Autodesk Inventor part; units mm, degrees
ref_plane "YZ Plane" through (0, 0, 0) normal (1, 0, 0) x (0, 1, 0)
ref_plane "XZ Plane" through (0, 0, 0) normal (0, 1, 0) x (-1, 0, 0)
ref_plane "XY Plane" through (0, 0, 0) normal (0, 0, 1) x (1, 0, 0)
sketch "Sketch1" plane through (0, 0, 0) normal (0, 1, 0) x (-1, 0, 0)
  line L0 (0, 0) -> (-2, 0)
  line L1 (-2, 0) -> (-4, 0)
  line L2 (0, 0) -> (0, -15)
  line L3 (0, -15) -> (0, -25)
  circle A0 centre (0, -25) radius 10
  line L4 (-1.5, -15.1131) -> (0, -15.1131)
  line L5 (0, -15.1131) -> (0, -15)
  line L6 (-1.5, -15) -> (-1.5, -15.1131)
  line L7 (-1.5, -15.1131) -> (-2, 0)
  line L8 (0, -15) -> (-1.5, -15)
  line L9 (-1.5, -15) -> (-2, -15)
  line L10 (-2, -15) -> (-2, -15.202)
  line L11 (-2, -15.202) -> (-4, 0)
  line L12 (0, -25) -> (0, -35)
  circle A1 centre (0, -25) radius 9.2
  line L13 (-1.5, -15.1131) -> (-1.4733, -15.9187)
  point P0 (0, -34.2)
  dimension "d7" = 18.4
  dimension "d2" = 15
  dimension "d4" = 10
  dimension "d6" = 0.5
  dimension "d10" = 1.5
  dimension "d11" = 2
  dimension "d12" = 2
revolve "Revolution1" add sketch "Sketch1" angle 180 about axis through (0, 0, 0) along (0, 0, 1) contours L7 L9 L10 L11 L1 | L7 A0 L10 L9 | L13 A1 L12 A0
sketch "Sketch2" plane through (0, 0, 0) normal (0, 0, 1) x (1, 0, 0)
  line L0 (5, 0) -> (-5, 0)
  line L1 (-14, 0) -> (14, 0)
  arc A0 (2, 0) -> (-2, 0) centre (0, 0) ccw
  line L2 (0, 0) -> (0, 16) construction
  line L3 (-10, 0) -> (10, 0)
  line L4 (10, 0) -> (10, 15)
  line L5 (10, 15) -> (-10, 15)
  line L6 (-10, 15) -> (-10, 0)
  point P0 (0, 0)
  point P1 (0, 0)
  point P2 (-10, 0)
  point P3 (10, 0)
  dimension "d29" = 20
  dimension "d33" = 15
  dimension "d34" = 15
extrude "Base" add sketch "Sketch2" along normal blind 7 contours L0 A0 L1 L6 L5 L4
sketch "Sketch3" plane through (0, 0, 0) normal (0, 0, -1) x (-1, 0, 0)
  line L0 (0, -3) -> (0, 18)
  line L1 (-10, 15) -> (10, 15)
  point P0 (0, 0)
  point P1 (0, 9.5)
  dimension "d30" = 5.5
hole "Screw Hole" at (0, 9.5, 0) direction (0, 0, 1) diameter 4.2 end through all counterbore diameter 8 counterbore depth 3
sketch "Sketch4" plane through (0, 0, 0) normal (0, 0, -1) x (-1, 0, 0)
  line L0 (-2, 0) -> (-10, 0)
  line L1 (0, 0) -> (0, -2) construction
  line L2 (6, 0) -> (6, 6)
  line L3 (6, 6) -> (8, 6)
  line L4 (6, 6) -> (4, 6)
  line L5 (4, 6) -> (5, 0)
  line L6 (7, 0) -> (8, 6)
  line L7 (7, 0) -> (5, 0)
  line L8 (10, 0) -> (2, 0)
  line L9 (6, 0) -> (6, 4)
  line L10 (7.6667, 4) -> (4.3333, 4)
  line L11 (0, 0) -> (0, 18)
  line L12 (10, 0) -> (4, 0)
  line L13 (-6, 0) -> (-6, 6)
  line L14 (-6, 6) -> (-8, 6)
  line L15 (-6, 6) -> (-4, 6)
  line L16 (-4, 6) -> (-5, 0)
  line L17 (-7, 0) -> (-8, 6)
  line L18 (-7, 0) -> (-5, 0)
  line L19 (-6, 0) -> (-6, 4)
  line L20 (-7.6667, 4) -> (-4.3333, 4)
  point P0 (5, 0)
  point P1 (-5, 0)
  point P2 (-5, 0)
extrude "Keyway" cut sketch "Sketch4" against normal through all contours L0 L13 L20 L16 | L0 L17 L20 L13 | L7 L5 L10 L2 | L2 L10 L6 L7
sketch "Sketch5" plane through (10, 0, 0) normal (1, 0, 0) x (0, 0, -1)
  line L0 (0, 15) -> (-7, 15)
  line L1 (0, 15) -> (-7, 15)
  line L2 (0, 0) -> (-7, 0)
  line L3 (-7, 15) -> (-7, 0)
  line L4 (-7, 15) -> (-7, 0)
  line L5 (-7, 0) -> (-6.5, 0)
  line L6 (-7, 15) -> (-6.5, 0)
  dimension "d37" = 0.5
extrude "Taper" cut sketch "Sketch5" against normal through all
fillet "Fillet1" radius 1 3 edges at (-10, 7.5, 0) (0, 15, 0) (10, 7.5, 0)
equation "\"d34\" = d33"
properties part number "markerWithRodEnd_3DPrint"
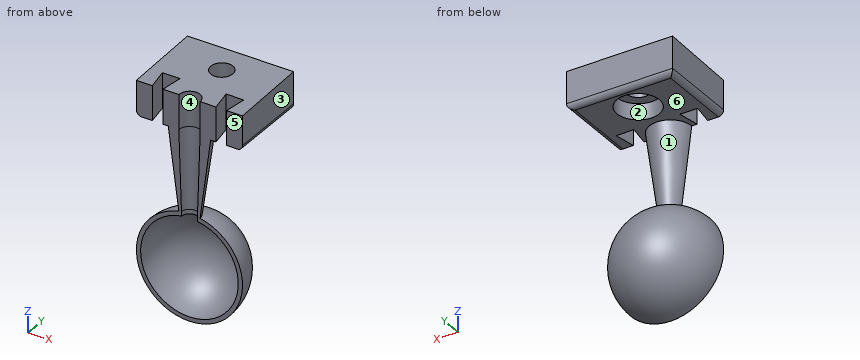
Design review of the part built by this model. Coordinates are the model's own, in mm. Face numbers are marked on the shaded views. A direction names the side the tool comes from. Give positions to 0.01 mm unless a question says otherwise; leave off trailing zeros. Loops run counter-clockwise (first coordinate to the right, second up) from the corner with the lowest first, then second, coordinate; pieces in that order, holes last. Notation, with made-up numbers: (76.5, 69) - (100.5, 69) arc R26 cw to (100.5, 83) - close; hole circle Ø1 at (66, 72). An arc over 180 degrees is marked (long way). Use CSV: the item, a comma, the result in double quotes. Start each with the question number.
1. Add section B-B (y = 12.5). State the section outline as (x, z) points, plus the area to 3 significant figures.
2. Machinability: for the marked faces 1, 2, 3 and 4, which of the approach directions +Z, -Z, +X, -X, +Y, -Y give a long, thin tool a straight path to every point of the face, cutting with its end or side? Answer none if there is none.
3. Draft analysis for pull direction Z (two halves, no side actions). For the marked faces 5 and 6, state which applies: released by +Z, released by -Z, zero draft, split by the parting line, or undercut.
4. Add section D-D (z = -27.5). State the section outline as (x, y) points, plus the area to 3 significant figures.
5. Add section C-C (z = 4). State the section outline as (x, y) points.
6. Add section A-A (x = 0). State the section outline as (y, z) points, plus the area to 3 significant figures.
7. Insertion check: P1, Ø6.5, axis at x = 0, y = 9.5, coming from the -Z side; P2, Ø3, axis at x = 1.5, y = 6, coming from the -Z side; P3, Ø6.5, axis at x = 0, y = 9.5, coming from the +Z side (3 decimals); P4, Ø1.5, axis at y = 11, z = -29, coming from the -X side. Each pin has a flat end and moves straight along its axis. Give the tip position at first contact, or say it passes through.
8. Wall thickness on L1, parallel to Y at x = 0, z = 5.9; L2, parallel to X at y = 9.5, z = 2; L3, parallel to X at y = 9.5, z = 6.05: over which ranges is each line inside the solid? List them lowest first.
Results found:
1,outline,"(-10, 1) arc R1 ccw to (-9, 0) - (-2.65, 0) - (-2.65, 3) - (2.65, 3) - (2.65, 0) - (9, 0) arc R1 ccw to (10, 1) - (10, 6.92) - (-10, 6.92) - close"
1,area,"122 mm²"
2,face 1,"+Y"
2,face 2,"none"
2,face 3,"+Z, -Z, +X, +Y, -Y"
2,face 4,"+Z, -Y"
3,face 5,"zero draft"
3,face 6,"undercut"
4,outline,"(-9.68, 0) - (-8.85, 0) arc R8.85 cw to (8.85, 0) - (9.68, 0) arc R9.68 ccw to start"
4,area,"24.1 mm²"
5,outline,"(-10, 0) - (-7, 0) - (-7.67, 4) - (-4.33, 4) - (-5, 0) - (-2, 0) arc R2 cw to (2, 0) - (5, 0) - (4.33, 4) - (7.67, 4) - (7, 0) - (10, 0) - (10, 15) - (-10, 15) - close; hole circle Ø4.2 at (0, 9.5)"
6,outline,"(0, -35) arc R10 ccw to (2, -15.2) - (4, 0) - (5.5, 0) - (5.5, 3) - (7.4, 3) - (7.4, 6.75) - (2, 6.57) - (2, 0) - (1.5, -15.11) - (1.47, -15.92) arc R9.2 cw to (0, -34.2) - close; (11.6, 3) - (13.5, 3) - (13.5, 0) - (14, 0) arc R1 ccw to (15, 1) - (15, 7) - (11.6, 6.89) - close"
6,area,"89.9 mm²"
7,P1,"stops at z = -32.81"
7,P2,"stops at z = -33.83"
7,P3,"stops at z = 6.925"
7,P4,"passes through"
8,L1,"y = 2 to 7.4, 11.6 to 15"
8,L2,"x = -10 to -4, 4 to 10"
8,L3,"x = -10 to -2.1, 2.1 to 10"
